Check sheet for the modelled part. Datum: model origin and axes. Units: mm. A direction names the side the tool comes from. Round coordinates to 2 decimals unless told otherwise and drop trailing zeros. Order: outer loops, then holes, each group sorted by start corner. A loop starts at its lowest first (then second) coordinate and runs counter-clockwise, first axis right, second up.
from build123d import *

# Parameters (mm, degrees)
ESQUISSE1_R             = 3
EXTRUSION1_DEPTH        = 8
ESQUISSE2_R             = 1
ENL_V_MAT_EXTRU_1_DEPTH = 9
ENL_V_MAT_EXTRU_4_DEPTH = 4
ESQUISSE4_R             = 2
ENL_V_MAT_EXTRU_5_DEPTH = 12
CHANFREIN1_SIZE         = 3


with BuildPart() as part:
    # Esquisse1 → Extrusion1 (new body)
    with BuildSketch(Plane.XY):
        Polygon((32, 6), (13, 6), (13, 11), (0, 11), (0, 0), (32, 0), align=None)
        with Locations((6, 5.5)):
            Circle(ESQUISSE1_R, mode=Mode.SUBTRACT)
    extrude(amount=EXTRUSION1_DEPTH)

    # Esquisse2 → Enlèv. mat.-Extru.1 (cut, through all)
    with BuildSketch(Plane.XY.offset(8)):
        with Locations((32, 3)):
            Circle(ESQUISSE2_R)
    extrude(amount=-ENL_V_MAT_EXTRU_1_DEPTH, mode=Mode.SUBTRACT)

    # Esquisse3 → Enlèv. mat.-Extru.4 (cut)
    with BuildSketch(Plane.XZ):
        Polygon((25, 0), (32, 4), (32, 0), align=None)
    extrude(amount=-ENL_V_MAT_EXTRU_4_DEPTH, mode=Mode.SUBTRACT)

    # Esquisse4 → Enlèv. mat.-Extru.5 (cut, through all)
    with BuildSketch(Plane.XZ):
        with Locations((20, 4)):
            Circle(ESQUISSE4_R)
    extrude(amount=-ENL_V_MAT_EXTRU_5_DEPTH, mode=Mode.SUBTRACT)

    # Chanfrein1
    chanfrein1_edges = [part.edges().sort_by_distance(p)[0] for p in [
        (0, 0, 4),
        (0, 11, 4),
    ]]
    chamfer(chanfrein1_edges, length=CHANFREIN1_SIZE)


solid = part.part
1) Draft check along X on faces 1 (the face through (16, 4, 8)), 2 (the face through (7.384, 2.838, 3.944)), 3 (the face through (28.5, 2, 2)). Enter one of: pulls with the +X half, pulls with the -X half, needs draft (parallel to the pull), parting line crosses it, or undercut.
2) Sectioned sample at B-B on z = 1. Record the cut outline in (x, y).
3) Sectioned sample at C-C on x = 6. Record the cut outline in (y, z).
4) Set-up check for faces 4 (the face through (12, 4, 0)), 5 (the face through (30, 4, 1)), 6 (the face through (23, 6, 4)): record each of +Z, -Z, +X, -X, +Y, -Y from which the full face is reachable in a straight line by a thin tool's end or side.
5) Gauge pin test, flat end, axial feed: pin 1 (4 mm diameter, centred on y = 9.5, z = 5, fed in from +X). Record the tip position at first contact, or that the pin passes through.
6) Sectioned sample at D-D on z = 3. Record the cut outline in (x, y), and give its area (3 significant figures).
7) Sectioned sample at A-A on y = 5.5. Record the cut outline in (x, z), and give its area (3 significant figures).
8) Scan lines: line 1 (Z direction, x = 20, y = 3.4); line 2 (Y direction, x = 6, z = 3.75); line 3 (Y direction, x = 18, z = 7.75). Record each from-to range of solid material in increasing order.
Values found:
1. face 1: needs draft
1. face 2: undercut
1. face 3: pulls with the +X half
2. outline: (0, 3) - (3, 0) - (26.75, 0) - (26.75, 4) - (32, 4) - (32, 6) - (13, 6) - (13, 11) - (3, 11) - (0, 8) - close; hole circle Ø6 at (6, 5.5)
3. outline: (0, 0) - (2.5, 0) - (2.5, 8) - (0, 8) - close; (8.5, 0) - (11, 0) - (11, 8) - (8.5, 8) - close
4. face 4: -Z, +X, -X, +Y, -Y
4. face 5: -Z, +X, -Y
4. face 6: +Z, -Z, +X, +Y
5. pin 1: stops at x = 13
6. outline: (0, 3) - (3, 0) - (18.27, 0) - (18.27, 6) - (13, 6) - (13, 11) - (3, 11) - (0, 8) - close; (21.73, 0) - (30.25, 0) - (30.25, 4) - (32, 4) - (32, 6) - (21.73, 6) - close; hole circle Ø6 at (6, 5.5)
6. area: 192 mm2
7. outline: (0, 0) - (3, 0) - (3, 8) - (0, 8) - close; (9, 0) - (32, 0) - (32, 8) - (9, 8) - close; hole circle Ø4 at (20, 4)
7. area: 195 mm2
8. line 1: z = 0 to 2, 6 to 8
8. line 2: y = 0 to 2.5, 8.5 to 11
8. line 3: y = 0 to 6
